from build123d import *

# Parameters (mm, degrees)
F0_W     = 109.8725795746
F0_H     = 96.4100509882
F1_DEPTH = 25.4
F3_D     = 4.2


with BuildPart() as f1:
    # F0 (on Top) → F1 (new body)
    with BuildSketch(Plane.XY):
        Rectangle(F0_W, F0_H)
    extrude(amount=F1_DEPTH)

    # F3 (through all)
    with Locations(Plane.XY.offset(25.4)):
        with Locations((-27.8564244509, -34.5673300326), (-15.4279861599, 14.1568621621), (5.9229629114, 8.01777374), (33.7983295321, 8.2835806534), (32.0603661239, -34.5673300326), (3.3077781554, -25.1481775194)):
            Hole(F3_D / 2)


solid = f1.part
Could you check a few things on this model? Use its own coordinates, in mm. Give positions to 0.01 mm unless a question says otherwise; leave off trailing zeros. Answer as a JSON object with one key per item and string values.
Q1. We'd pull the mould along X, two halves only. Please class faces 1 (the flat face through (-1, 1, 25.4)), 2 (the flat face through (54.936, -1, 13)), 3 (the cylindrical face through (33.727, -35.845, 12.522)): released by +X, released by -X, zero draft, split by the parting line, or undercut.
Taken from the geometry:
{"face 1": "zero draft", "face 2": "released by +X", "face 3": "undercut"}
Q2. Please list where these lines run through material, in increasing order: L1, parallel to X at y = -25, z = 23.75; L2, parallel to Y at x = 4, z = 14; L3, parallel to X at y = 9, z = 8.
Taken from the geometry:
{"L1": "x = -54.94 to 1.21, 5.4 to 54.94", "L2": "y = -48.21 to -27.13, -23.17 to 7.17, 8.86 to 48.21", "L3": "x = -54.94 to 4.07, 7.78 to 31.82, 35.77 to 54.94"}
Q3. Will these pins go through, and if not, where does the flat tip stop? pin 1 Ø5 at (x, y) = (5.92, 8.02) entering from +Z; pin 2 Ø2.5 at (x, y) = (-27.86, -34.57) entering from -Z.
Taken from the geometry:
{"pin 1": "stops at z = 25.4", "pin 2": "passes through"}
